from build123d import *

# Parameters (mm, degrees)
F0_R      = 5
F1_DEPTH  = 21.5
F2_R      = 6.05
F3_DEPTH  = 1.8
F4_R      = 5.45
F5_DEPTH  = 1.2
F6_R      = 6.05
F7_DEPTH  = 3.95
F8_R      = 4.525
F9_DEPTH  = 3
F10_R     = 6.05
F11_DEPTH = 22.45
F12_R     = 4.525
F13_DEPTH = 2.75
F14_R     = 6.05
F15_DEPTH = 3.95
F16_R     = 5.5
F17_DEPTH = 1.25
F18_R     = 6.05
F19_DEPTH = 1.4


with BuildPart() as f1:
    # F0 (on Top) → F1 (new body)
    with BuildSketch(Plane.XY):
        Circle(F0_R)
    extrude(amount=-F1_DEPTH)

    # F2 (on Top) → F3 (join)
    with BuildSketch(Plane.XY):
        Circle(F2_R)
    extrude(amount=F3_DEPTH)

    # F4 (on face) → F5 (join)
    with BuildSketch(Plane.XY.offset(1.8)):
        Circle(F4_R)
    extrude(amount=F5_DEPTH)

    # F6 (on face) → F7 (join)
    with BuildSketch(Plane.XY.offset(3)):
        Circle(F6_R)
    extrude(amount=F7_DEPTH)

    # F8 (on face) → F9 (join)
    with BuildSketch(Plane.XY.offset(6.95)):
        Circle(F8_R)
    extrude(amount=F9_DEPTH)

    # F10 (on face) → F11 (join)
    with BuildSketch(Plane.XY.offset(9.95)):
        Circle(F10_R)
    extrude(amount=F11_DEPTH)

    # F12 (on face) → F13 (join)
    with BuildSketch(Plane.XY.offset(32.4)):
        Circle(F12_R)
    extrude(amount=F13_DEPTH)

    # F14 (on face) → F15 (join)
    with BuildSketch(Plane.XY.offset(35.15)):
        Circle(F14_R)
    extrude(amount=F15_DEPTH)

    # F16 (on face) → F17 (join)
    with BuildSketch(Plane.XY.offset(39.1)):
        Circle(F16_R)
    extrude(amount=F17_DEPTH)

    # F18 (on face) → F19 (join)
    with BuildSketch(Plane.XY.offset(40.35)):
        Circle(F18_R)
    extrude(amount=F19_DEPTH)


solid = f1.part
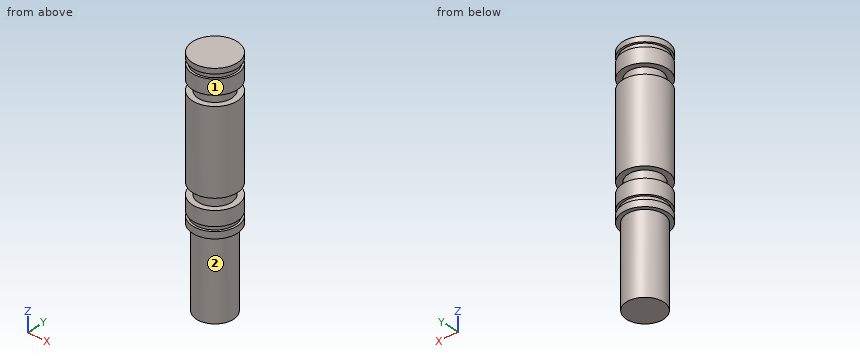
CAD build for the part. Positions are in the model's coordinates, mm. Face numbers are marked on the shaded views. A direction names the side the tool comes from. Give positions to 0.01 mm unless a question says otherwise; leave off trailing zeros. Loops run counter-clockwise (first coordinate to the right, second up) from the corner with the lowest first, then second, coordinate; pieces in that order, holes last. Notation, with made-up numbers: M 73.5,47.25 L 100.5,47.25 A35 cw 100.5,80.25 Z; hole C 6.25,68.25 d7. An arc over 180 degrees is marked long. Answer in a Markdown table with one row per item. Add a question column.
Item 1: Probe probe 1 along Z at (x, y) = (-0.75, -5); probe 2 along Z at (x, y) = (0, 4.75); probe 3 along Z at (x, y) = (5.75, 1.25). List the from-to ranges inside material, lowest first.
Item 2: Band-saw the part on A-A on z = -14.5. Give the cut face in (x, y).
Item 3: Band-saw the part on B-B on z = 29.5. Give the cut face in (x, y), then the cut area to 3 significant figures.
Item 4: Tool access for the marked faces 1 and 2: list every direction of +Z, -Z, +X, -X, +Y, -Y with a clear straight run to the whole face (end or side of a thin tool).
Item 5: Drop flat-ended pins along their axis: P1, Ø1.5, axis at y = -4, z = 15, coming from the +X side; P2, Ø1, axis at x = 4, z = 6, coming from the +Y side; P3, Ø4, axis at x = -0.5, z = 33, coming from the -Y side; P4, Ø6, axis at x = -3, z = 8.5, coming from the +Y side. Give the stop position or say it passes through.
Reply:
| question | item | result |
|---|---|---|
| 1 | probe 1 | z = 0 to 6.95, 9.95 to 32.4, 35.15 to 41.75 |
| 1 | probe 2 | z = -21.5 to 6.95, 9.95 to 32.4, 35.15 to 41.75 |
| 1 | probe 3 | z = 0 to 1.8, 3 to 6.95, 9.95 to 32.4, 35.15 to 39.1, 40.35 to 41.75 |
| 2 | outline | C 0,0 d10 |
| 3 | outline | C 0,0 d12.1 |
| 3 | area | 115 mm^2 |
| 4 | face 1 | +Z, -Z |
| 4 | face 2 | -Z |
| 5 | P1 | stops at x = 5.1 |
| 5 | P2 | stops at y = 4.93 |
| 5 | P3 | stops at y = -6.05 |
| 5 | P4 | stops at y = 6.04 |
